```python
from build123d import *

# Parameters (mm, degrees)
SKETCH1_W           = 22.0472
SKETCH1_H           = 27.686
BOSS_EXTRUDE1_DEPTH = 28.8036
SKETCH2_W           = 14.732
SKETCH2_H           = 5.6388
BOSS_EXTRUDE2_DEPTH = 3.048
SKETCH3_R           = 11.0236
BOSS_EXTRUDE3_DEPTH = 8.0772
SKETCH4_R           = 9.525
CUT_EXTRUDE1_DEPTH  = 6.35
FILLET1_R           = 1.27
FILLET2_R           = 0.762
SKETCH5_R           = 1.143
CUT_EXTRUDE2_DEPTH  = 2.54


with BuildPart() as part:
    # Sketch1 → Boss-Extrude1 (new body)
    with BuildSketch(Plane(origin=(0, 0, 0), x_dir=(1, 0, 0), z_dir=(0, 1, 0))):
        with Locations((11.0236, 13.843)):
            Rectangle(SKETCH1_W, SKETCH1_H)
    extrude(amount=BOSS_EXTRUDE1_DEPTH)

    # Sketch2 → Boss-Extrude2 (add)
    with BuildSketch(Plane.XY):
        with Locations((11.0236, 20.8026)):
            Rectangle(SKETCH2_W, SKETCH2_H)
    extrude(amount=BOSS_EXTRUDE2_DEPTH)

    # Sketch3 → Boss-Extrude3 (add)
    with BuildSketch(Plane(origin=(0, 28.8036, 0), x_dir=(1, 0, 0), z_dir=(0, 1, 0))):
        with Locations((11.0236, 16.637)):
            Circle(SKETCH3_R)
    extrude(amount=BOSS_EXTRUDE3_DEPTH)

    # Sketch4 → Cut-Extrude1 (cut)
    with BuildSketch(Plane(origin=(0, 36.8808, 0), x_dir=(1, 0, 0), z_dir=(0, 1, 0))):
        with Locations((11.0236, 36.2966)):
            Circle(SKETCH4_R)
        with Locations((28.049313028, 26.4668)):
            Circle(SKETCH4_R)
        with Locations((28.049313028, 6.8072)):
            Circle(SKETCH4_R)
        with Locations((11.0236, -3.0226)):
            Circle(SKETCH4_R)
        with Locations((-6.002113028, 6.8072)):
            Circle(SKETCH4_R)
        with Locations((-6.002113028, 26.4668)):
            Circle(SKETCH4_R)
    extrude(amount=-CUT_EXTRUDE1_DEPTH, mode=Mode.SUBTRACT)

    # Fillet1
    fillet1_edges = [part.edges().sort_by_distance(p)[0] for p in [
        (0, 14.4018, -27.686),
        (22.0472, 14.4018, -27.686),
        (22.0472, 14.4018, 0),
        (0, 14.4018, 0),
    ]]
    fillet(fillet1_edges, radius=FILLET1_R)

    # Fillet2
    fillet2_edges = [part.edges().sort_by_distance(p)[0] for p in [
        (18.3896, 17.9832, 1.524),
        (18.3896, 23.622, 1.524),
        (3.6576, 23.622, 1.524),
        (3.6576, 17.9832, 1.524),
    ]]
    fillet(fillet2_edges, radius=FILLET2_R)

    # Sketch5 → Cut-Extrude2 (cut)
    with BuildSketch(Plane.XY.offset(3.048)):
        with Locations((6.5786, 20.8026)):
            Circle(SKETCH5_R)
        with Locations((15.4686, 20.8026)):
            Circle(SKETCH5_R)
    extrude(amount=-CUT_EXTRUDE2_DEPTH, mode=Mode.SUBTRACT)


solid = part.part
```
Read the model definition and answer for the solid it produces. Units are mm, in the model's axes. A direction names the side the tool comes from. Round coordinates to 2 decimals unless told otherwise and drop trailing zeros. Write each loop counter-clockwise with the first axis right and the second up, starting at its lowest first coordinate (ties: lowest second). Pieces come first, ordered by that corner, then holes. Notation, with made-up numbers: (43.5, 60) -> (69.5, 60) arc R28 cw to (69.5, 80) -> close; hole circle Ø9 at (86.25, 10.5). An arc over 180 degrees is marked (long way). Answer in a Markdown table with one row per item. Add a question column.
1) Consider line 1 (Y direction, x = 6.5, z = 1); line 2 (Z direction, x = 10, y = 13); line 3 (Y direction, x = 18.25, z = -4.5). Determine where each line is inside the solid, lowest interval first.
2) Find section A-A, the plane y = 28. Determine the outline of the cut face in (x, z).
3) Determine the mould class of faces 1 (the face through (0.36, 14.6, -27.3)), 2 (the face through (10.98, 33.75, -26.77)), 3 (the face through (2, 30.531, -22)), 4 (the face through (0.01, 31.89, -17.12)) for opening direction X: pulls with the +X half, pulls with the -X half, needs draft (parallel to the pull), parting line crosses it, or undercut.
4) Given P1, Ø0.9, axis at y = 21.5, z = 2, coming from the +X side; P2, Ø0.9, axis at x = 14, z = 1, coming from the +Y side; P3, Ø2.5, axis at x = 9.5, z = 2, coming from the -Y side, each flat-ended and moving along its own axis, determine where each tip first touches the part or whether it passes through.
5) Which of the six approach directions +Z, -Z, +X, -X, +Y, -Y give full straight-line access (tool end or side, diameter ignored) to faces 5 (the face through (18.39, 21, 2)), 6 (the face through (19.822, 33.75, -11.606)), 7 (the face through (5.74, 21.58, 1.8))?
6) Find section C-C, the plane z = -20.5. Determine the outline of the cut face in (x, y), and give its area (3 significant figures).
7) Find section D-D, the plane x = 2.25. Determine the outline of the cut face in (y, z).
8) Find section B-B, the plane x = 13.5. Determine the outline of the cut face in (y, z), and give its area (3 significant figures).
Findings below:
| question | item | result |
|---|---|---|
| 1 | line 1 | 17.98 to 19.66, 21.94 to 23.62 |
| 1 | line 2 | -27.69 to 0 |
| 1 | line 3 | 0 to 28.8 |
| 2 | outline | (0, -26.42) arc R1.27 ccw to (1.27, -27.69) -> (20.78, -27.69) arc R1.27 ccw to (22.05, -26.42) -> (22.05, -1.27) arc R1.27 ccw to (20.78, 0) -> (1.27, 0) arc R1.27 ccw to (0, -1.27) -> close |
| 3 | face 1 | pulls with the -X half |
| 3 | face 2 | undercut |
| 3 | face 3 | needs draft |
| 3 | face 4 | parting line crosses it |
| 4 | P1 | x = 18.39 |
| 4 | P2 | y = 23.62 |
| 4 | P3 | y = 17.98 |
| 5 | face 5 | +Z, +X, +Y, -Y |
| 5 | face 6 | +Z, +X, +Y |
| 5 | face 7 | +Z |
| 6 | outline | (0, 0) -> (22.05, 0) -> (22.05, 28.8) -> (21.35, 28.8) -> (21.35, 30.53) -> (20.62, 30.53) -> (20.62, 36.88) -> (1.42, 36.88) -> (1.42, 30.53) -> (0.7, 30.53) -> (0.7, 28.8) -> (0, 28.8) -> close |
| 6 | area | 793 mm² |
| 7 | outline | (0, -27.69) -> (28.8, -27.69) -> (28.8, -23.31) -> (30.53, -23.31) -> (30.53, -21.71) -> (36.88, -21.71) -> (36.88, -11.56) -> (30.53, -11.56) -> (30.53, -9.96) -> (28.8, -9.96) -> (28.8, 0) -> (0, 0) -> close |
| 8 | outline | (0, -27.69) -> (28.8, -27.69) -> (28.8, -27.38) -> (30.53, -27.38) -> (30.53, -27.1) -> (36.88, -27.1) -> (36.88, -6.17) -> (30.53, -6.17) -> (30.53, -5.9) -> (28.8, -5.9) -> (28.8, 0) -> (23.62, 0) -> (23.62, 3.05) -> (17.98, 3.05) -> (17.98, 0) -> (0, 0) -> close |
| 8 | area | 985 mm² |
